from build123d import *

# Parameters (mm, degrees)
CUT_EXTRUDE2_DEPTH      = 460.620517828
CUT_EXTRUDE2_DEPTH_BACK = 460.620517828
CUT_EXTRUDE3_DEPTH      = 476.132634543
CUT_EXTRUDE3_DEPTH_BACK = 476.132634543
SKETCH3_R               = 50


with BuildPart() as part:
    # Sketch1 → Revolve1 (revolve)
    with BuildSketch(Plane(origin=(0, 0, 0), x_dir=(1, 0, 0), z_dir=(0, 1, 0)), mode=Mode.PRIVATE) as revolve1_sk:
        with BuildLine():
            Line((-212.857142857, 80), (-232.857142857, 80))
            Line((-232.857142857, 80), (-232.857142857, 120))
            Line((-232.857142857, 120), (307.142857143, 120))
            ThreePointArc((307.142857143, 120), (391.995670885, 84.852813742), (427.142857143, 0))
            Line((427.142857143, 0), (307.142857143, 0))
            Line((307.142857143, 0), (187.142857143, 0))
            Line((187.142857143, 0), (187.142857143, 100))
            Line((187.142857143, 100), (-212.857142857, 100))
            Line((-212.857142857, 100), (-212.857142857, 80))
        make_face()
    revolve(revolve1_sk.sketch.rotate(Axis((-156.292678098, 0, 0), (1, 0, 0)), 180), axis=Axis((-156.292678098, 0, 0), (1, 0, 0)))

    # Sketch2 → Cut-Extrude2 (cut, two sides: drawn at the far end of the back side and taken through both)
    with BuildSketch(Plane.XY.offset(-CUT_EXTRUDE2_DEPTH_BACK)):
        Polygon((525.404105683, 50), (227.142857143, 50), (227.142857143, 120), (587.948795726, 120), (587.948795726, -120), (227.142857143, -120), (227.142857143, -50), (525.404105683, -50), align=None)
    extrude(amount=CUT_EXTRUDE2_DEPTH + CUT_EXTRUDE2_DEPTH_BACK, mode=Mode.SUBTRACT)

    # Sketch3 → Cut-Extrude3 (cut, two sides: drawn at the far end of the back side and taken through both)
    with BuildSketch(Plane(origin=(0, 50, 0), x_dir=(1, 0, 0), z_dir=(0, 1, 0)).offset(-CUT_EXTRUDE3_DEPTH_BACK)):
        with Locations(Location((307.142857143, 0, 0), (0, 0, 180))):
            Circle(SKETCH3_R)
    extrude(amount=CUT_EXTRUDE3_DEPTH + CUT_EXTRUDE3_DEPTH_BACK, mode=Mode.SUBTRACT)


solid = part.part
Geometry: final body of the model. Coordinates: model frame, mm. A direction names the side the tool comes from. Give positions to 0.01 mm unless a question says otherwise; leave off trailing zeros. Loops run counter-clockwise (first coordinate to the right, second up) from the corner with the lowest first, then second, coordinate; pieces in that order, holes last. Notation, with made-up numbers: M -38,-25 L 13,-25 A15 ccw 13,-5 Z; hole C 62.5,87 d6. An arc over 180 degrees is marked long. Put each result on its own line as item: value. Start each with the question number.
1) Ray query, line 1 along Y through (x, z) = (58, 0); line 2 along X through (y, z) = (-87, -12); line 3 along Y through (x, z) = (-221, 0). Return the intervals inside material, ascending.
2) Cut plane B-B (y = -25). Output: boundary loops of the cut face in (x, z), then the cut area to 3 significant figures.
3) Pull-direction query (X, two-part tool) for faces 4 (the cylindrical face through (-15.66, -30.04, 95.38)), 5 (the flat face through (-232.857, 78, -25)), 6 (the flat face through (227.143, -78, -2)), 7 (the flat face through (-212.857, -67, -45)); classes: pulls with the +X half, pulls with the -X half, needs draft (parallel to the pull), parting line crosses it, or undercut.
4) Contact query for flat-ended pins moving along their axis: pin 1 (8 mm diameter, centred on x = -113, z = -83.5, fed in from -Y); pin 2 (1 mm diameter, centred on y = -39.5, z = -61.5, fed in from -X); pin 3 (12 mm diameter, centred on x = 338, y = 36.5, fed in from +Z). Output: stop coordinate, or through.
5) Cut plane D-D (z = 66). Output: boundary loops of the cut face in (x, y).
6) Cut plane C-C (x = -26). Output: boundary loops of the cut face in (y, z), then the cut area to 3 significant figures.
7) Access query for faces 1 (the flat face through (323, 50, -50)), 2 (the flat face through (320, -50, -50)), 3 (the cylindrical face through (-222.997, -3.517, -79.923)). Directions: +Z, -Z, +X, -X, +Y, -Y. A direction counts if a zero-diameter tool reaches every point of the face in a straight line with its end or side. Return the directions, or none.
8) Cut plane A-A (z = 0). Output: boundary loops of the cut face in (x, y).
Verdict:
1. line 1: -120 to -100, 100 to 120
1. line 2: -232.86 to -212.86, 187.14 to 227.14
1. line 3: -120 to -80, 80 to 120
2. outline: M -232.86,-117.37 L 307.14,-117.37 A117.37 ccw 307.14,117.37 L -232.86,117.37 L -232.86,75.99 L -212.86,75.99 L -212.86,96.82 L 187.14,96.82 L 187.14,-96.82 L -212.86,-96.82 L -212.86,-75.99 L -232.86,-75.99 Z; hole C 307.14,0 d100
2. area: 60,000 mm2
3. face 4: undercut
3. face 5: pulls with the -X half
3. face 6: pulls with the +X half
3. face 7: undercut
4. pin 1: y = -89.89
4. pin 2: x = 187.14
4. pin 3: z = 112.49
5. outline: M -232.86,-100.22 L 227.14,-100.22 L 227.14,-50 L 394,-50 A100.22 ccw 394,50 L 227.14,50 L 227.14,100.22 L -232.86,100.22 L -232.86,45.21 L -212.86,45.21 L -212.86,75.13 L 187.14,75.13 L 187.14,-75.13 L -212.86,-75.13 L -212.86,-45.21 L -232.86,-45.21 Z
6. outline: C 0,0 d240; hole C 0,0 d200
6. area: 13,800 mm2
7. face 1: +Z, -Z, +X, +Y
7. face 2: +Z, -Z, +X, -Y
7. face 3: -X
8. outline: M -232.86,-120 L 227.14,-120 L 227.14,-50 L 257.14,-50 L 257.14,50 L 227.14,50 L 227.14,120 L -232.86,120 L -232.86,80 L -212.86,80 L -212.86,100 L 187.14,100 L 187.14,-100 L -212.86,-100 L -212.86,-80 L -232.86,-80 Z; M 357.14,-50 L 416.23,-50 A120 ccw 416.23,50 L 357.14,50 Z
